from build123d import *

# Parameters (mm, degrees)
F0_R     = 62.5
F0_R_2   = 4.5
F0_W     = 18
F0_H     = 18
F1_DEPTH = 20
F2_R     = 30
F2_W     = 18
F2_H     = 18
F3_DEPTH = 2
F4_R     = 30
F4_W     = 18
F4_H     = 18
F5_DEPTH = 2
F6_R     = 4.5
F7_DEPTH = 30


with BuildPart() as f1:
    # F0 (on Front) → F1 (new body)
    with BuildSketch(Plane.XZ):
        Circle(F0_R)
        with Locations((-33.587572, -33.587572)):
            Circle(F0_R_2, mode=Mode.SUBTRACT)
        with Locations((33.587572, -33.587572)):
            Circle(F0_R_2, mode=Mode.SUBTRACT)
        with Locations((-33.587572, 33.587572)):
            Circle(F0_R_2, mode=Mode.SUBTRACT)
        Rectangle(F0_W, F0_H, mode=Mode.SUBTRACT)
        with Locations((33.587572, 33.587572)):
            Circle(F0_R_2, mode=Mode.SUBTRACT)
    extrude(amount=F1_DEPTH)

    # F2 (on face) → F3 (join)
    with BuildSketch(Plane(origin=(0, 0, 0), x_dir=(-1, 0, 0), z_dir=(0, 1, 0))):
        Circle(F2_R)
        Rectangle(F2_W, F2_H, mode=Mode.SUBTRACT)
    extrude(amount=F3_DEPTH)

    # F4 (on face) → F5 (join)
    with BuildSketch(Plane.XZ.offset(20)):
        Circle(F4_R)
        Rectangle(F4_W, F4_H, mode=Mode.SUBTRACT)
    extrude(amount=F5_DEPTH)

    # F6 (on face) → F7 (cut)
    with BuildSketch(Plane.XZ.offset(22)):
        with Locations((0, 22.5)):
            Circle(F6_R)
        with Locations((22.5, 0)):
            Circle(F6_R)
        with Locations((0, -22.5)):
            Circle(F6_R)
        with Locations((-22.5, 0)):
            Circle(F6_R)
    extrude(amount=-F7_DEPTH, mode=Mode.SUBTRACT)


solid = f1.part
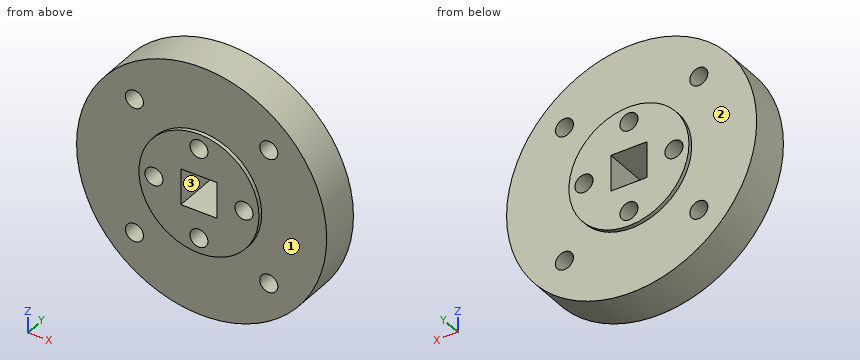
Geometry: final body of the model. Coordinates: model frame, mm. Face numbers are marked on the shaded views. A direction names the side the tool comes from. Give positions to 0.01 mm unless a question says otherwise; leave off trailing zeros. Write each loop counter-clockwise with the first axis right and the second up, starting at its lowest first coordinate (ties: lowest second). Pieces come first, ordered by that corner, then holes. Notation, with made-up numbers: (12, 18) -> (28, 18) arc R33 ccw to (28, 49) -> close; hole circle Ø7 at (23, 35.25). An arc over 180 degrees is marked (long way). Answer as a JSON object with one key per item and string values.
1. Cut plane D-D on z = 22.5. Output: boundary loops of the cut face in (x, y).
Ans:
{"outline": "(-58.31, -20) -> (-19.84, -20) -> (-19.84, -22) -> (-4.5, -22) -> (-4.5, 2) -> (-19.84, 2) -> (-19.84, 0) -> (-58.31, 0) -> close; (4.5, -22) -> (19.84, -22) -> (19.84, -20) -> (58.31, -20) -> (58.31, 0) -> (19.84, 0) -> (19.84, 2) -> (4.5, 2) -> close"}
2. Access query for the marked faces 1, 2 and 3. Directions: +Z, -Z, +X, -X, +Y, -Y. A direction counts if a zero-diameter tool reaches every point of the face in a straight line with its end or side. Return the directions, or none.
Ans:
{"face 1": "-Y", "face 2": "+Y", "face 3": "+Y, -Y"}
3. Ray query, probe 1 along X at (y, z) = (-5, -3.5); probe 2 along X at (y, z) = (-5.75, 37.5); probe 3 along X at (y, z) = (-11.25, -34). Return the intervals inside material, ascending. Write a range as from..to.
Ans:
{"probe 1": "x = -62.4..-25.33, -19.67..-9, 9..19.67, 25.33..62.4", "probe 2": "x = -50..-35.81, -31.36..31.36, 35.81..50", "probe 3": "x = -52.44..-38.07, -29.11..29.11, 38.07..52.44"}
4. Cut plane B-B on x = -22.5. Output: boundary loops of the cut face in (y, z), and give its area (3 significant figures).
Ans:
{"outline": "(-22, -19.84) -> (-20, -19.84) -> (-20, -58.31) -> (0, -58.31) -> (0, -19.84) -> (2, -19.84) -> (2, -4.5) -> (-22, -4.5) -> close; (-22, 4.5) -> (2, 4.5) -> (2, 19.84) -> (0, 19.84) -> (0, 58.31) -> (-20, 58.31) -> (-20, 19.84) -> (-22, 19.84) -> close", "area": "2,280 mm^2"}
5. Cut plane A-A on z = 0. Output: boundary loops of the cut face in (x, y), and give its area (3 significant figures).
Ans:
{"outline": "(-62.5, -20) -> (-30, -20) -> (-30, -22) -> (-27, -22) -> (-27, 2) -> (-30, 2) -> (-30, 0) -> (-62.5, 0) -> close; (-18, -22) -> (-9, -22) -> (-9, 2) -> (-18, 2) -> close; (9, -22) -> (18, -22) -> (18, 2) -> (9, 2) -> close; (27, -22) -> (30, -22) -> (30, -20) -> (62.5, -20) -> (62.5, 0) -> (30, 0) -> (30, 2) -> (27, 2) -> close", "area": "1,880 mm^2"}
6. Contact query for flat-ended pins moving along their axis: pin 1 (10.5 mm diameter, centred on x = 33.59, z = -33.59, fed in from -Y); pin 2 (2 mm diameter, centred on y = -18, z = 16, fed in from -X); pin 3 (3 mm diameter, centred on y = -9, z = 5.5, fed in from -X). Output: stop coordinate, or through.
Ans:
{"pin 1": "stops at y = -20", "pin 2": "stops at x = -60.67", "pin 3": "stops at x = -62.37"}
7. Cut plane C-C on x = 0. Output: boundary loops of the cut face in (y, z).
Ans:
{"outline": "(-22, -30) -> (-20, -30) -> (-20, -62.5) -> (0, -62.5) -> (0, -30) -> (2, -30) -> (2, -27) -> (-22, -27) -> close; (-22, -18) -> (2, -18) -> (2, -9) -> (-22, -9) -> close; (-22, 9) -> (2, 9) -> (2, 18) -> (-22, 18) -> close; (-22, 27) -> (2, 27) -> (2, 30) -> (0, 30) -> (0, 62.5) -> (-20, 62.5) -> (-20, 30) -> (-22, 30) -> close"}
